from build123d import *

# Parameters (mm, degrees)
ESQUISSE1_W             = 24.7
ESQUISSE1_H             = 24.7
BOSS_EXTRU_1_DEPTH      = 3.08
CHANFREIN1_SIZE         = 3
CONG_1_R                = 0.2
ESQUISSE2_W             = 6
ESQUISSE2_H             = 2.88
ENL_V_MAT_EXTRU_1_DEPTH = 22.08
ENL_V_MAT_EXTRU_2_DEPTH = 2.88


with BuildPart() as part:
    # Esquisse1 → Boss.-Extru.1 (new body)
    with BuildSketch(Plane(origin=(0, 0, 0), x_dir=(1, 0, 0), z_dir=(0, 1, 0))):
        with Locations((12.35, 12.35)):
            Rectangle(ESQUISSE1_W, ESQUISSE1_H)
    extrude(amount=BOSS_EXTRU_1_DEPTH)

    # Chanfrein1
    chanfrein1_edges = [part.edges().sort_by_distance(p)[0] for p in [
        (0, 1.54, -24.7),
        (24.7, 1.54, -24.7),
        (24.7, 1.54, 0),
        (0, 1.54, 0),
    ]]
    chamfer(chanfrein1_edges, length=CHANFREIN1_SIZE)

    # Congé1
    cong_1_edges = [part.edges().sort_by_distance(p)[0] for p in [
        (0, 3.08, -12.35),
        (12.35, 3.08, -24.7),
        (12.35, 3.08, 0),
        (24.7, 3.08, -12.35),
        (1.5, 3.08, -1.5),
        (23.2, 3.08, -1.5),
        (23.2, 3.08, -23.2),
        (1.5, 3.08, -23.2),
    ]]
    fillet(cong_1_edges, radius=CONG_1_R)

    # Esquisse2 → Enlèv. mat.-Extru.1 (cut)
    with BuildSketch(Plane(origin=(0, 0, -24.7), x_dir=(-1, 0, 0), z_dir=(0, 0, -1))):
        with Locations((-12.35, 1.44)):
            Rectangle(ESQUISSE2_W, ESQUISSE2_H)
    extrude(amount=-ENL_V_MAT_EXTRU_1_DEPTH, mode=Mode.SUBTRACT)

    # Esquisse3 → Enlèv. mat.-Extru.2 (cut)
    with BuildSketch(Plane.XZ):
        Polygon((3.124264069, -24.4), (21.575735931, -24.4), (24.4, -21.575735931), (24.4, -3.124264069), (21.575735931, -0.3), (3.124264069, -0.3), (0.3, -3.124264069), (0.3, -21.575735931), align=None)
    extrude(amount=-ENL_V_MAT_EXTRU_2_DEPTH, mode=Mode.SUBTRACT)


solid = part.part
Design review of the part built by this model. Coordinates are the model's own, in mm. A direction names the side the tool comes from. Give positions to 0.01 mm unless a question says otherwise; leave off trailing zeros. Loops run counter-clockwise (first coordinate to the right, second up) from the corner with the lowest first, then second, coordinate; pieces in that order, holes last. Notation, with made-up numbers: (-15, 65.25) -> (6, 65.25) arc R21 cw to (6, 94.25) -> close; hole circle Ø3 at (53, 13). An arc over 180 degrees is marked (long way). One line per question, with ' | ' between items. Start each with the question number.
(1) We need section A-A (y = 2.05). State the section outline as (x, z) points.
(2) Insertion check: P1, Ø8, axis at x = 9, z = -14.5, coming from the -Y side. The pin has a flat end and moves straight along its axis. Give the tip position at first contact, or say it passes through.
(3) For faces 5 (the face through (24.7, 1, -12)), 6 (the face through (6, 1, -24.4)), list the 3-axis set-ups (+Z, -Z, +X, -X, +Y, -Y) from which the entire face can be reached by the end or side of a thin tool; tool diameter is ignored.
(4) We need section B-B (z = -11.25). State the section outline as (x, y) points.
(5) We need section C-C (x = 4.25). State the section outline as (y, z) points, and give its area (3 significant figures).
(6) For line 1 (Z direction, x = 4, y = 1.9); line 2 (X direction, y = 1.35, z = -7.5); line 3 (Y direction, x = 9.5, z = -23.5), list the stretches that pass through material, from the lowest coordinate up.
(7) Draft analysis for pull direction X (two halves, no side actions). For faces 1 (the face through (12, 1, -0.3)), 2 (the face through (18, 1, -24.7)), 3 (the face through (23.2, 1.4, -1.5)), 4 (the face through (1.56, 3.02, -23.18)), state which applies: +X half, -X half, draft (parallel to the pull), parting line (faces both ways), or undercut.
The answers:
1) outline: (0, -21.7) -> (3, -24.7) -> (9.35, -24.7) -> (9.35, -24.4) -> (3.12, -24.4) -> (0.3, -21.58) -> (0.3, -3.12) -> (3.12, -0.3) -> (21.58, -0.3) -> (24.4, -3.12) -> (24.4, -21.58) -> (21.58, -24.4) -> (15.35, -24.4) -> (15.35, -24.7) -> (21.7, -24.7) -> (24.7, -21.7) -> (24.7, -3) -> (21.7, 0) -> (3, 0) -> (0, -3) -> close
2) P1: stops at y = 2.88
3) face 5: +Z, -Z, +X, +Y, -Y | face 6: -Y
4) outline: (0, 0) -> (0.3, 0) -> (0.3, 2.88) -> (24.4, 2.88) -> (24.4, 0) -> (24.7, 0) -> (24.7, 2.88) arc R0.2 ccw to (24.5, 3.08) -> (0.2, 3.08) arc R0.2 ccw to (0, 2.88) -> close
5) outline: (0, -24.7) -> (2.88, -24.7) arc R0.2 ccw to (3.08, -24.5) -> (3.08, -0.2) arc R0.2 ccw to (2.88, 0) -> (0, 0) -> (0, -0.3) -> (2.88, -0.3) -> (2.88, -24.4) -> (0, -24.4) -> close | area: 6.65 mm^2
6) line 1: z = -24.7 to -24.4, -0.3 to 0 | line 2: x = 0 to 0.3, 24.4 to 24.7 | line 3: y = 2.88 to 3.08
7) face 1: undercut | face 2: draft | face 3: +X half | face 4: -X half
